from build123d import *

# Parameters (mm, degrees)
SKETCH_1_W          = 50
SKETCH_1_H          = 30
EXTRUDE_1_DEPTH     = 10
EXTRUDE_2_DEPTH     = 10
SKETCH_3_R          = 5
CUT_EXTRUDE_1_DEPTH = 3
FILLET_1_R          = 3
FILLET_2_R          = 1


with BuildPart() as part:
    # 스케치1 → 보스-돌출1 (new body)
    with BuildSketch(Plane.XY):
        Rectangle(SKETCH_1_W, SKETCH_1_H)
    extrude(amount=EXTRUDE_1_DEPTH)

    # 스케치2 → 보스-돌출2 (add, symmetric)
    with BuildSketch(Plane(origin=(0, 0, 0), x_dir=(0, 0, -1), z_dir=(1, 0, 0))):
        Polygon((0, 0), (24.201197656, -24.201197656), (24.201197656, -29.201197656), (-14.510049854, -29.201197656), (-14.510049854, -24.201197656), (19.201197656, -24.201197656), (0, -5), align=None)
    extrude(amount=EXTRUDE_2_DEPTH, both=True)

    # 스케치3 → 컷-돌출1 (cut)
    with BuildSketch(Plane.XY.offset(10)):
        with Locations((-10, 0)):
            Circle(SKETCH_3_R)
    extrude(amount=-CUT_EXTRUDE_1_DEPTH, mode=Mode.SUBTRACT)

    # 필렛1
    fillet_1_edges = [part.edges().sort_by_distance(p)[0] for p in [
        (0, -15, 10),
        (0, -15, 0),
        (0, 15, 0),
        (25, -15, 5),
        (-25, -15, 5),
        (-25, 15, 5),
        (25, 15, 5),
        (0, 15, 10),
    ]]
    fillet(fillet_1_edges, radius=FILLET_1_R)

    # 필렛2
    fillet_2_edges = [part.edges().sort_by_distance(p)[0] for p in [
        (-10, -14.600598828, -9.600598828),
        (-10, -24.201197656, -2.345573901),
        (0, -24.201197656, -19.201197656),
        (-10, -26.701197656, 14.510049854),
        (0, -24.201197656, 14.510049854),
        (0, -29.201197656, 14.510049854),
        (0, -29.201197656, -24.201197656),
        (0, -24.201197656, -24.201197656),
        (10, -14.600598828, -9.600598828),
        (10, -24.201197656, -2.345573901),
        (10, -26.701197656, 14.510049854),
    ]]
    fillet(fillet_2_edges, radius=FILLET_2_R)


solid = part.part
Here's how the part is built. I have some questions about the finished solid (model axes, mm). A direction names the side the tool comes from. Coordinates: 2 decimals unless noted, no trailing zeros. Loops run counter-clockwise (first coordinate to the right, second up) from the corner with the lowest first, then second, coordinate; pieces in that order, holes last. Notation, with made-up numbers: (26, 43.5) -> (70, 43.5) arc R5 ccw to (70, 47.5) -> close; hole circle Ø1 at (-6.75, 29.5). An arc over 180 degrees is marked (long way). Use one line per item in the form item = value. Start each with the question number.
(1) If we section it at C-C (x = -17.5): Please give me the cut outline in (y, z), then the cut area to 3 significant figures.
(2) If we section it at B-B (y = -1.5): Please give me the cut outline in (x, z).
(3) On a 3-axis mill with a long thin cutter (end or side, diameter ignored), from which of +Z, -Z, +X, -X, +Y, -Y can I reach the whole of each face in a straight line? I mean faces 5 (the face through (-10, -26, -8)), 6 (the face through (10, -26, -8)), 7 (the face through (9.699, -13.064, -8.468)), 8 (the face through (0, 0, 10)). Say none if no direction works.
(4) We'd pull the mould along Z, two halves only. Please class faces 1 (the face through (0, -26, -24.201)), 2 (the face through (0, -29.201, -5)), 3 (the face through (0.35, -14.14, 0.9)), 4 (the face through (-9.715, -13.053, -8.479)): pulls with the +Z half, pulls with the -Z half, needs draft (parallel to the pull), parting line crosses it, or undercut.
(5) Will these pins go through, and if not, where does the flat tip stop? pin 1 (8 mm diameter, centred on x = 6.5, y = -5.5, fed in from +Z); pin 2 (4 mm diameter, centred on y = -14.5, z = -14, fed in from -X); pin 3 (7 mm diameter, centred on x = 9, y = -5, fed in from -Z).
(6) Please list where these lines run through material, in increasing order: line 1 along Y through (x, z) = (3, -8); line 2 along Y through (x, z) = (-2, 13); line 3 along Y through (x, z) = (6.5, 8).
(7) If we section it at A-A (x = 4.5): Please give me the cut outline in (y, z), then the cut area to 3 significant figures.
Verdict:
q1.outline = (-15, 3) arc R3 ccw to (-12, 0) -> (12, 0) arc R3 ccw to (15, 3) -> (15, 7) arc R3 ccw to (12, 10) -> (-12, 10) arc R3 ccw to (-15, 7) -> close
q1.area = 292 mm²
q2.outline = (-25, 0) -> (-10, 0) -> (-10, -1.5) -> (10, -1.5) -> (10, 0) -> (25, 0) -> (25, 10) -> (-5.23, 10) -> (-5.23, 7) -> (-14.77, 7) -> (-14.77, 10) -> (-25, 10) -> close
q3.face_5 = -Z, -X, -Y
q3.face_6 = -Z, +X, -Y
q3.face_7 = +X
q3.face_8 = +Z, +X, -X, +Y
q4.face_1 = pulls with the -Z half
q4.face_2 = needs draft
q4.face_3 = undercut
q4.face_4 = undercut
q5.pin_1 = 10
q5.pin_2 = -10
q5.pin_3 = -8.5
q6.line_1 = -29.2 to -24.2, -13 to -8
q6.line_2 = -29.2 to -24.2
q6.line_3 = -29.2 to -24.2, -14.83 to 14.83
q7.outline = (-29.2, -23.2) arc R1 ccw to (-28.2, -24.2) -> (-24.62, -24.2) arc R1 ccw to (-23.91, -23.91) -> (0, 0) -> (12, 0) arc R3 ccw to (15, 3) -> (15, 7) arc R3 ccw to (12, 10) -> (-12, 10) arc R3 ccw to (-15, 7) -> (-15, 3) arc R3 ccw to (-12, 0) -> (-5, 0) -> (-22.49, -17.49) arc R1 cw to (-24.2, -16.79) -> (-24.2, 13.51) arc R1 ccw to (-25.2, 14.51) -> (-28.2, 14.51) arc R1 ccw to (-29.2, 13.51) -> close
q7.area = 595 mm²
